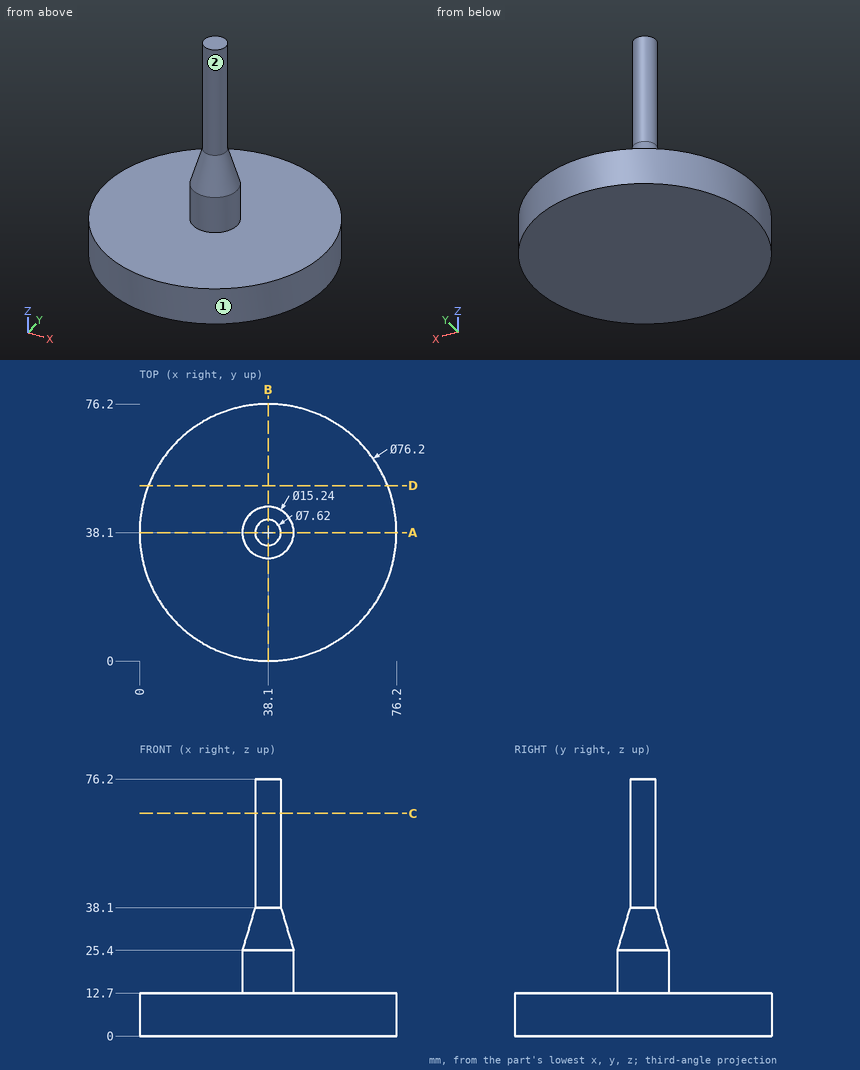
Part print with two shaded views. Sizes in mm from the minimum x, y, z corner. A direction names the side the tool comes from. Give positions to 0.01 mm unless a question says otherwise; leave off trailing zeros. Order: outer loops, then holes, each group sorted by start corner. A loop starts at its lowest first (then second) coordinate and runs counter-clockwise, first axis right, second up. Notation, with made-up numbers: M 49,80.5 L 66,80.5 A20 cw 66,98.5 Z; hole C 47,7.5 d1. An arc over 180 degrees is marked long. Write item = value, one per line.
Q1. Flat gauge pins, fed straight in: pin 1 (4 mm diameter, centred on x = 55, y = 32.5, fed in from +Z); pin 2 (12 mm diameter, centred on y = 19.5, z = 21.5, fed in from -X); pin 3 (4 mm diameter, centred on y = 34.5, z = 34, fed in from -X). Where does each tip first touch, or does it go through?
Derived:
pin_1 = 12.7
pin_2 = through
pin_3 = 33.08
Q2. Cut at A-A, the plane y = 38.1. List the corners of the cut face in (x, z).
Derived:
outline = M 0,0 L 76.2,0 L 76.2,12.7 L 45.72,12.7 L 45.72,25.4 L 41.91,38.1 L 41.91,76.2 L 34.29,76.2 L 34.29,38.1 L 30.48,25.4 L 30.48,12.7 L 0,12.7 Z
Q3. Tool access for the marked faces 1 and 2: list every direction of +Z, -Z, +X, -X, +Y, -Y with a clear straight run to the whole face (end or side of a thin tool).
Derived:
face_1 = +Z, -Z
face_2 = +Z
Q4. Cut at C-C, the plane z = 66. List the corners of the cut face in (x, y).
Derived:
outline = C 38.1,38.1 d7.62
Q5. Cut at D-D, the plane y = 52. List the corners of the cut face in (x, z).
Derived:
outline = M 2.63,0 L 73.57,0 L 73.57,12.7 L 2.63,12.7 Z
Q6. Drill centre lines: line 1 (Z direction, x = 35, y = 64); line 2 (X direction, y = 38.5, z = 48); line 3 (X direction, y = 35.5, z = 15). Where is each one in solid material? Low to high. Write a range as [from, to].
Derived:
line_1 = [0, 12.7]
line_2 = [34.31, 41.89]
line_3 = [30.94, 45.26]
